Work out the finished part from the listing and answer in its coordinate system (mm). Face numbers are marked on the shaded views. A direction names the side the tool comes from. Coordinates: 2 decimals unless noted, no trailing zeros. Order: outer loops, then holes, each group sorted by start corner. A loop starts at its lowest first (then second) coordinate and runs counter-clockwise, first axis right, second up.
1. The part is cut by section B-B, the plane z = 11. Give the vertices of the cut face in (x, y), then the cut area to 3 significant figures.
2. The part is cut by section A-A, the plane x = 0. Give the vertices of the cut face in (y, z), then the cut area to 3 significant figures.
3. Flat-ended cylindrical pins translate along their axes: pin 1 Ø12 at (x, z) = (-4, 45.5) entering from -Y; pin 2 Ø10 at (y, z) = (1.5, 30.5) entering from +X; pin 3 Ø3 at (x, z) = (-5.5, 15) entering from -Y. Find the tip coordinate at first contact, or state that the pin passes through.
4. Find the intervals of material crossed by probe 1 along Z at (x, y) = (10.5, 1.75); probe 2 along Y at (x, z) = (-0.75, 36); probe 3 along X at (y, z) = (-0.5, 33), in increasing order.
5. A tool of negligible diameter and unlimited length cuts with its end or side. For the marked faces 1 and 2, from which of +Z, -Z, +X, -X, +Y, -Y can it reach the whole face along a straight path? Write none if from no direction.
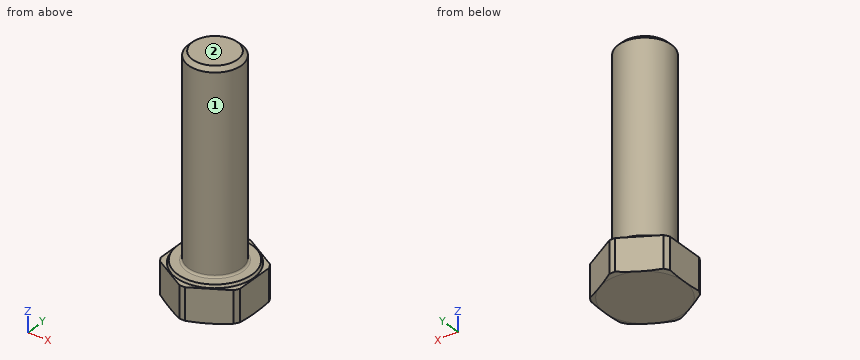
Autodesk Inventor part; units mm, degrees
ref_plane "DP402_XY" through (0, 6.773, 60) normal (1, 0, 0) x (0, 0, -1)
ref_plane "DP402_YZ" through (0, 6.773, 60) normal (0, 0, -1) x (0, 1, 0)
ref_plane "DP402_ZX" through (0, 6.773, 60) normal (0, 1, 0) x (1, 0, 0)
sketch "Sketch_3" plane through (0, 0, 0) normal (1, 0, 0) x (0, 0, -1)
  line L0 (10.8, 0) -> (-60, 0)
  line L1 (-60, 0) -> (-60, 6.773)
  line L2 (-60, 6.773) -> (-58.773, 8)
  line L3 (-58.773, 8) -> (-0.6, 8)
  arc A0 (-0.6, 8) -> (0, 8.6) centre (-0.6, 8.6) ccw
  line L4 (0, 8.6) -> (0, 11.25)
  line L5 (0, 11.25) -> (0.8, 11.7)
  line L6 (0.8, 11.7) -> (0.8, 13.38)
  line L7 (0.8, 13.38) -> (10.4302, 13.38)
  line L8 (10.4302, 13.38) -> (10.8, 12)
  line L9 (10.8, 12) -> (10.8, 0)
  line L10 (10.8, 0) -> (-60, 0)
revolve "Revolution1" add sketch "Sketch_3" angle 360 about axis through (0, 0, -10.8) along (0, 0, -1)
thread "Thread1"
sketch "Sketch_1" plane through (0, 0, 0) normal (0, 0, 1) x (1, 0, 0)
  line L0 (-24, -24) -> (24, -24)
  line L1 (24, -24) -> (24, 24)
  line L2 (24, 24) -> (-24, 24)
  line L3 (-24, 24) -> (-24, -24)
  line L4 (-12, -6.9282) -> (0, -13.8564)
  line L5 (0, -13.8564) -> (12, -6.9282)
  line L6 (12, -6.9282) -> (12, 6.9282)
  line L7 (12, 6.9282) -> (0, 13.8564)
  line L8 (0, 13.8564) -> (-12, 6.9282)
  line L9 (-12, 6.9282) -> (-12, -6.9282)
extrude "Extrusion1" cut sketch "Sketch_1" against normal blind 10.8
ref_plane "DP402_XY" through (0, 6.773, 60) normal (1, 0, 0) x (0, 0, -1)
ref_plane "DP402_YZ" through (0, 6.773, 60) normal (0, 0, -1) x (0, 1, 0)
ref_plane "DP402_ZX" through (0, 6.773, 60) normal (0, 1, 0) x (1, 0, 0)
ref_plane "DPG1_XY" through (0, 8, 58.773) normal (1, 0, 0) x (0, 0, -1)
ref_plane "DPG1_YZ" through (0, 8, 58.773) normal (0, 0, -1) x (0, 1, 0)
ref_plane "DPG1_ZX" through (0, 8, 58.773) normal (0, 1, 0) x (1, 0, 0)
ref_plane "DPG2_XY" through (0, -8, 58.773) normal (1, 0, 0) x (0, 0, -1)
ref_plane "DPG2_YZ" through (0, -8, 58.773) normal (0, 0, -1) x (0, 1, 0)
ref_plane "DPG2_ZX" through (0, -8, 58.773) normal (0, 1, 0) x (1, 0, 0)
ref_plane "SCHRAUBE_XY" through (0, 0, 0) normal (0, 0, -1) x (1, 0, 0)
ref_plane "SCHRAUBE_YZ" through (0, 0, 0) normal (1, 0, 0) x (0, -1, 0)
ref_plane "SCHRAUBE_ZX" through (0, 0, 0) normal (0, -1, 0) x (0, 0, -1)
properties part number "SLZ_63_Schraube_M16x60#"
Geometry says:
1. outline: circle Ø16 at (0, 0)
1. area: 201 mm2
2. outline: (-13.38, -10.43) - (-12, -10.8) - (12, -10.8) - (13.38, -10.43) - (13.38, -0.8) - (11.7, -0.8) - (11.25, 0) - (8.6, 0) arc R0.6 cw to (8, 0.6) - (8, 58.77) - (6.77, 60) - (-6.77, 60) - (-8, 58.77) - (-8, 0.6) arc R0.6 cw to (-8.6, 0) - (-11.25, 0) - (-11.7, -0.8) - (-13.38, -0.8) - close
2. area: 1,240 mm2
3. pin 1: stops at y = -8
3. pin 2: stops at x = 8
3. pin 3: stops at y = -6.93
4. probe 1: z = -10.8 to 0
4. probe 2: y = -7.96 to 7.96
4. probe 3: x = -7.98 to 7.98
5. face 1: +Z
5. face 2: +Z, +X, -X, +Y, -Y
